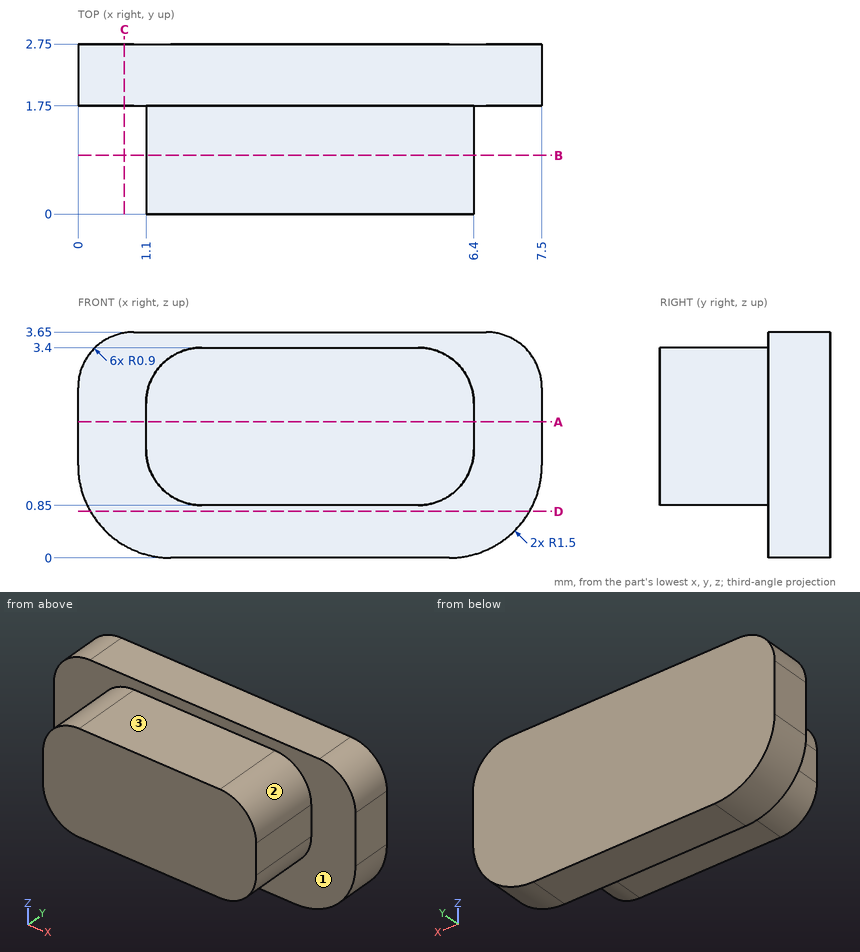
Input: dimensioned drawing with shaded views. Units: mm. Origin: part minimum x, y, z. A direction names the side the tool comes from. Coordinates: 2 decimals unless noted, no trailing zeros. Loops run counter-clockwise (first coordinate to the right, second up) from the corner with the lowest first, then second, coordinate; pieces in that order, holes last.
Q1. Contact query for flat-ended pins moving along their axis: pin 1 (0.6 mm diameter, centred on y = 1, z = 2, fed in from -X); pin 2 (0.8 mm diameter, centred on y = 1, z = 2, fed in from +X); pin 3 (1.4 mm diameter, centred on x = 4, y = 1, fed in from +Z). Output: stop coordinate, or through.
Results are:
pin 1: stops at x = 1.1
pin 2: stops at x = 6.4
pin 3: stops at z = 3.4
Q2. Section C-C, the plane x = 0.75. Return the cut outline in (y, z).
Results are:
outline: (1.75, 0.2) - (2.75, 0.2) - (2.75, 3.64) - (1.75, 3.64) - close
Q3. Set-up query: the marked faces 1, 2 and 3. Return all of +Z, -Z, +X, -X, +Y, -Y with unobstructed straight access to the full face (end or side cutting, diameter ignored); none if empty.
Results are:
face 1: -Y
face 2: +Z, +X, -Y
face 3: +Z, +X, -X, -Y
Q4. Section D-D, the plane z = 0.75. Return the cut outline in (x, y), and give its area (3 significant figures).
Results are:
outline: (0.2, 1.75) - (7.3, 1.75) - (7.3, 2.75) - (0.2, 2.75) - close
area: 7.10 mm2
Q5. Section B-B, the plane y = 0.95. Return the cut outline in (x, z).
Results are:
outline: (1.1, 1.75) arc R0.9 ccw to (2, 0.85) - (5.5, 0.85) arc R0.9 ccw to (6.4, 1.75) - (6.4, 2.5) arc R0.9 ccw to (5.5, 3.4) - (2, 3.4) arc R0.9 ccw to (1.1, 2.5) - close
Q6. Section A-A, the plane z = 2.2. Return the cut outline in (x, y).
Results are:
outline: (0, 1.75) - (1.1, 1.75) - (1.1, 0) - (6.4, 0) - (6.4, 1.75) - (7.5, 1.75) - (7.5, 2.75) - (0, 2.75) - close
Q7. Line query: line 1 along Z through (x, y) = (2, 0.4); line 2 along X through (y, z) = (0.55, 2.15); line 3 along Y through (x, z) = (4, 0.7). Output: solid intervals per line, ascending.
Results are:
line 1: z = 0.85 to 3.4
line 2: x = 1.1 to 6.4
line 3: y = 1.75 to 2.75
